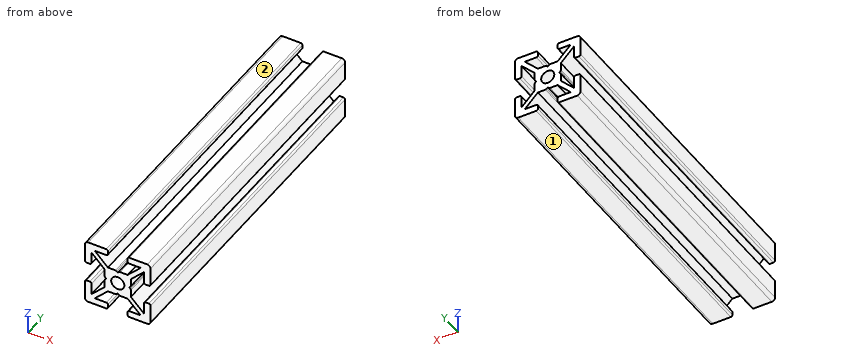
from build123d import *

# Parameters (mm, degrees)
SKETCH1_R           = 2
BOSS_EXTRUDE1_DEPTH = 100
FILLET1_R           = 1
FILLET2_R           = 0.5
FILLET4_R           = 0.5


with BuildPart() as part:
    # Sketch1 → Boss-Extrude1 (new body)
    with BuildSketch(Plane(origin=(0, 0, 0), x_dir=(1, 0, 0), z_dir=(0, 1, 0))):
        Polygon((7, 18), (7, 20), (0, 20), (0, 13), (2, 13), (2, 17), (6, 13), (6, 10.5), (6.5, 10), (6, 9.5), (6, 7), (2, 3), (2, 7), (0, 7), (0, 0), (7, 0), (7, 2), (3, 2), (7, 6), (9.5, 6), (10, 6.5), (10.5, 6), (13, 6), (17, 2), (13, 2), (13, 0), (20, 0), (20, 7), (18, 7), (18, 3), (14, 7), (14, 9.5), (13.5, 10), (14, 10.5), (14, 13), (18, 17), (18, 13), (20, 13), (20, 20), (13, 20), (13, 18), (17, 18), (13, 14), (10.5, 14), (10, 13.5), (9.5, 14), (7, 14), (3, 18), align=None)
        with Locations((10, 10)):
            Circle(SKETCH1_R, mode=Mode.SUBTRACT)
    extrude(amount=BOSS_EXTRUDE1_DEPTH)

    # Fillet1
    fillet1_edges = [part.edges().sort_by_distance(p)[0] for p in [
        (0, 50, -20),
        (20, 50, -20),
        (20, 50, 0),
        (0, 50, 0),
    ]]
    fillet(fillet1_edges, radius=FILLET1_R)

    # Fillet2
    fillet2_edges = [part.edges().sort_by_distance(p)[0] for p in [
        (2, 50, -13),
        (0, 50, -13),
        (7, 50, -20),
        (7, 50, -18),
        (13, 50, -18),
        (13, 50, -20),
        (20, 50, -13),
        (18, 50, -13),
        (18, 50, -7),
        (20, 50, -7),
        (13, 50, 0),
        (13, 50, -2),
        (7, 50, -2),
        (7, 50, 0),
        (0, 50, -7),
        (2, 50, -7),
    ]]
    fillet(fillet2_edges, radius=FILLET2_R)

    # Fillet4
    fillet4_edges = [part.edges().sort_by_distance(p)[0] for p in [
        (9.5, 50, -14),
        (10.5, 50, -14),
        (14, 50, -10.5),
        (14, 50, -9.5),
        (10.5, 50, -6),
        (9.5, 50, -6),
        (6, 50, -9.5),
        (6, 50, -10.5),
    ]]
    fillet(fillet4_edges, radius=FILLET4_R)


solid = part.part
CAD build for the part. Positions are in the model's coordinates, mm. Face numbers are marked on the shaded views. Coordinates: 2 decimals unless noted, no trailing zeros. Loops run counter-clockwise (first coordinate to the right, second up) from the corner with the lowest first, then second, coordinate; pieces in that order, holes last. Notation, with made-up numbers: (60, 88.25) - (89, 88.25) arc R23 ccw to (89, 112.25) - close; hole circle Ø9 at (33.25, -10.75). An arc over 180 degrees is marked (long way). Use one line per item in the form item = value. Start each with the question number.
1) Flat gauge pins, fed straight in: pin 1 (1.5 mm diameter, centred on x = 10, y = 69, fed in from -Z); pin 2 (0.7 mm diameter, centred on y = 57.5, z = -11.5, fed in from -X); pin 3 (2.5 mm diameter, centred on x = 10, z = -10, fed in from +Y); pin 4 (0.7 mm diameter, centred on x = 12.5, y = 27.5, fed in from +Z). Where does each tip first touch, or does it go through?
2) Two-plate mould, pull along Z, no slides. Class the marked faces 1 and 2: +Z half, -Z half, draft (parallel to the pull), parting line (faces both ways), or undercut.
3) Band-saw the part on A-A (z = -15.75). Give the cut face in (x, y), and give its area (3 significant figures).
4) Band-saw the part on B-B (x = 4.5). Give the cut face in (y, z), and give its area (3 significant figures).
5) Drill centre lines: L1, parallel to Z at x = 10, y = 51.5; L2, parallel to X at y = 46, z = -10; L3, parallel to X at y = 70, z = -16.5. Where is each one in solid material? Low to high. Write a range as from..to.
Check values:
q1.pin_1 = -14
q1.pin_2 = 6
q1.pin_3 = through
q1.pin_4 = -6
q2.face_1 = -Z half
q2.face_2 = +Z half
q3.outline = (0, 0) - (2, 0) - (2, 100) - (0, 100) - close; (3.25, 0) - (5.25, 0) - (5.25, 100) - (3.25, 100) - close; (14.75, 0) - (16.75, 0) - (16.75, 100) - (14.75, 100) - close; (18, 0) - (20, 0) - (20, 100) - (18, 100) - close
q3.area = 800 mm2
q4.outline = (0, -20) - (100, -20) - (100, -18) - (0, -18) - close; (0, -16.5) - (100, -16.5) - (100, -14.5) - (0, -14.5) - close; (0, -5.5) - (100, -5.5) - (100, -3.5) - (0, -3.5) - close; (0, -2) - (100, -2) - (100, 0) - (0, 0) - close
q4.area = 800 mm2
q5.L1 = -13.5..-12, -8..-6.5
q5.L2 = 6.5..8, 12..13.5
q5.L3 = 0..2, 2.5..4.5, 15.5..17.5, 18..20
